Verification items for the finished model (mm, model axes). Face numbers are marked on the shaded views. A direction names the side the tool comes from. Coordinates: 2 decimals unless noted, no trailing zeros. Write each loop counter-clockwise with the first axis right and the second up, starting at its lowest first coordinate (ties: lowest second). Pieces come first, ordered by that corner, then holes. Notation, with made-up numbers: (1.5, 50) -> (60.5, 50) arc R6 ccw to (60.5, 58) -> close; hole circle Ø4 at (-20, 88.5). An arc over 180 degrees is marked (long way). Answer in a Markdown table with one row per item.
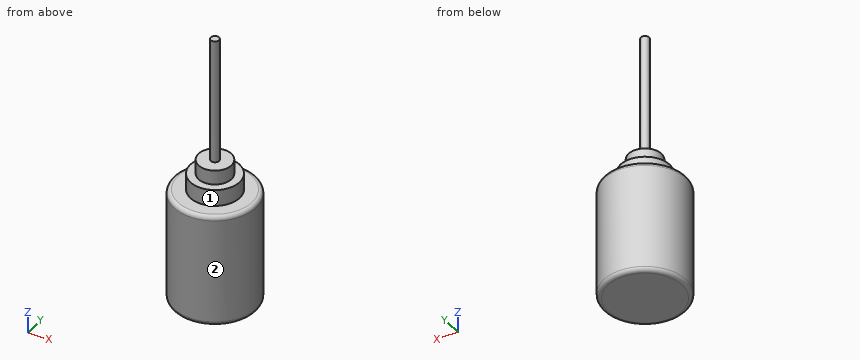
```python
from build123d import *

# Parameters (mm, degrees)
SKETCH1_R           = 20
SKETCH1_R_2         = 2
BOSS_EXTRUDE1_DEPTH = 55
SKETCH1_3_R         = 2
BOSS_EXTRUDE2_DEPTH = 131
SKETCH2_R           = 8
BOSS_EXTRUDE3_DEPTH = 15
SKETCH3_R           = 12
BOSS_EXTRUDE4_DEPTH = 8
FILLET1_R           = 2
SCALE1_SCALE        = 0.5
SCALE2_SCALE        = 0.5
SCALE3_SCALE        = 1.25


with BuildPart() as part:
    # Sketch1 → Boss-Extrude1 (new body)
    with BuildSketch(Plane.XY):
        Circle(SKETCH1_R)
        Circle(SKETCH1_R_2, mode=Mode.SUBTRACT)
    extrude(amount=BOSS_EXTRUDE1_DEPTH)

    # Sketch1<3> → Boss-Extrude2 (add)
    with BuildSketch(Plane.XY):
        Circle(SKETCH1_3_R)
    extrude(amount=BOSS_EXTRUDE2_DEPTH)

    # Sketch2 → Boss-Extrude3 (add)
    with BuildSketch(Plane.XY.offset(55)):
        Circle(SKETCH2_R)
    extrude(amount=BOSS_EXTRUDE3_DEPTH)

    # Sketch3 → Boss-Extrude4 (add)
    with BuildSketch(Plane.XY.offset(55)):
        Circle(SKETCH3_R)
    extrude(amount=BOSS_EXTRUDE4_DEPTH)

    # Fillet1
    fillet1_edges = [part.edges().sort_by_distance(p)[0] for p in [
        (-20, 0, 55),
        (-20, 0, 0),
    ]]
    fillet(fillet1_edges, radius=FILLET1_R)


with BuildPart() as part_1:
    # Scale1: scaled about (0, 0, 30.5101534)
    add(part.part.scale(SCALE1_SCALE).moved(Location((0, 0, 15.2550767))))


with BuildPart() as part_2:
    # Scale2: scaled about (0, 0, 30.5101534)
    add(part_1.part.scale(SCALE2_SCALE).moved(Location((0, 0, 15.2550767))))


with BuildPart() as part_3:
    # Scale3: scaled about (0, 0, 30.5101534)
    add(part_2.part.scale(SCALE3_SCALE).moved(Location((0, 0, -7.62753835))))


solid = part_3.part
```
1. Tool access check on the marked faces 1 and 2. Record the directions out of +Z, -Z, +X, -X, +Y, -Y that give a thin tool (end or side, any length) a straight path to the whole face; none if there is none.
Geometry says:
| item | result |
|---|---|
| face 1 | +Z |
| face 2 | +Z, -Z |
2. Section check C-C, the plane z = 30. Record the boundary of the cut face in (x, y), plus the area to 3 significant figures.
Geometry says:
| item | result |
|---|---|
| outline | circle Ø12.5 at (0, 0) |
| area | 123 mm^2 |
3. Section check A-A, the plane x = 0. Record the boundary of the cut face in (y, z) (3 decimals).
Geometry says:
| item | result |
|---|---|
| outline | (-6.25, 21.601) arc R0.625 ccw to (-5.625, 20.976) -> (5.625, 20.976) arc R0.625 ccw to (6.25, 21.601) -> (6.25, 37.538) arc R0.625 ccw to (5.625, 38.163) -> (3.75, 38.163) -> (3.75, 40.663) -> (2.5, 40.663) -> (2.5, 42.851) -> (0.625, 42.851) -> (0.625, 61.913) -> (-0.625, 61.913) -> (-0.625, 42.851) -> (-2.5, 42.851) -> (-2.5, 40.663) -> (-3.75, 40.663) -> (-3.75, 38.163) -> (-5.625, 38.163) arc R0.625 ccw to (-6.25, 37.538) -> close |
4. Depth check by flat-ended pin: P1, Ø2, axis at y = 1.5, z = 28, coming from the +X side; P2, Ø1, axis at y = -2.5, z = 29.5, coming from the +X side; P3, Ø4, axis at x = 2, z = 57, coming from the -Y side (3 decimals). Enter the tip coordinate at first touch or a pass-through.
Geometry says:
| item | result |
|---|---|
| P1 | x = 6.23 |
| P2 | x = 5.92 |
| P3 | y = -0.625 |
5. Thickness scan on line 1 (Z direction, x = 0, y = -1.25); line 2 (Z direction, x = -4.75, y = -0.25); line 3 (X direction, y = -2, z = 32.5). Record the ranges inside material, lowest first. Write a range as from..to.
Geometry says:
| item | result |
|---|---|
| line 1 | 20.98..42.85 |
| line 2 | 20.98..38.16 |
| line 3 | -5.92..5.92 |
